```python
from build123d import *

# Parameters (mm, degrees)
BOSS_EXTRUDE1_DEPTH = 10
SKETCH2_R           = 12.5
CUT_EXTRUDE1_DEPTH  = 271.924343683
SKETCH3_R           = 7.5
CUT_EXTRUDE2_DEPTH  = 10


with BuildPart() as part:
    # Sketch1 → Boss-Extrude1 (new body)
    with BuildSketch(Plane.XY):
        with BuildLine():
            Line((-20, 0), (-20, 250))
            ThreePointArc((-20, 250), (0, 270), (20, 250))
            Line((20, 250), (20, 0))
            ThreePointArc((20, 0), (0, -20), (-20, 0))
        make_face()
    extrude(amount=BOSS_EXTRUDE1_DEPTH)

    # Sketch2 → Cut-Extrude1 (cut, through all)
    with BuildSketch(Plane(origin=(0, 0, 0), x_dir=(-1, 0, 0), z_dir=(0, 0, -1))):
        Circle(SKETCH2_R)
        with Locations((0, 250)):
            Circle(SKETCH2_R)
    extrude(amount=-CUT_EXTRUDE1_DEPTH, mode=Mode.SUBTRACT)

    # Sketch3 → Cut-Extrude2 (cut)
    with BuildSketch(Plane(origin=(0, 0, 0), x_dir=(-1, 0, 0), z_dir=(0, 0, -1))):
        with Locations((0, 125)):
            Circle(SKETCH3_R)
    extrude(amount=-CUT_EXTRUDE2_DEPTH, mode=Mode.SUBTRACT)


solid = part.part
```
Could you check a few things on this model? Use its own coordinates, in mm. Give positions to 0.01 mm unless a question says otherwise; leave off trailing zeros. Loops run counter-clockwise (first coordinate to the right, second up) from the corner with the lowest first, then second, coordinate; pieces in that order, holes last. Notation, with made-up numbers: (-12.75, 6.25) - (13.25, 6.25) arc R20 ccw to (13.25, 23.25) - close; hole circle Ø9 at (41.5, 87). An arc over 180 degrees is marked (long way). Answer in a Markdown table with one row per item. Add a question column.
Q1. If we section it at C-C (z = 5): List the corners of the cut face in (x, y) for me, plus the area to 3 significant figures.
Q2. Please list where these lines run through material, in increasing order: L1, parallel to Y at x = 0, z = 2.5; L2, parallel to Y at x = -5, z = 1.5; L3, parallel to Y at x = -9, z = 8.5. Write a range as from..to.
Q3. If we section it at B-B (y = 125): List the corners of the cut face in (x, z) for me.
Q4. For pin 1 (5 mm diameter, centred on x = 14, z = 4, fed in from +Y); pin 2 (1 mm diameter, centred on x = 11, z = 5.5, fed in from -Y); pin 3 (2 mm diameter, centred on x = 15.5, z = 6, fed in from +Y) (3 decimals), each with a flat end and sliding along its axis, tell me the tip position at first contact or that it passes through.
Q5. If we section it at A-A (x = 0): List the corners of the cut face in (y, z) for me, plus the area to 3 significant figures.
Q6. If we section it at D-D (x = -17.5): List the corners of the cut face in (y, z) for me.
Q7. We'd pull the mould along Y, two halves only. Please class faces 1 (the face through (0, -20, 5)), 2 (the face through (0, 270, 5)), 3 (the face through (-11.923, 3.755, 4.93)): +Y half, -Y half, draft (parallel to the pull), parting line (faces both ways), or undercut.
The answers:
| question | item | result |
|---|---|---|
| 1 | outline | (-20, 0) arc R20 ccw to (20, 0) - (20, 250) arc R20 ccw to (-20, 250) - close; hole circle Ø25 at (0, 0); hole circle Ø25 at (0, 250); hole circle Ø15 at (0, 125) |
| 1 | area | 10,100 mm^2 |
| 2 | L1 | y = -20..-12.5, 12.5..117.5, 132.5..237.5, 262.5..270 |
| 2 | L2 | y = -19.36..-11.46, 11.46..119.41, 130.59..238.54, 261.46..269.36 |
| 2 | L3 | y = -17.86..-8.67, 8.67..241.33, 258.67..267.86 |
| 3 | outline | (-20, 0) - (-7.5, 0) - (-7.5, 10) - (-20, 10) - close; (7.5, 0) - (20, 0) - (20, 10) - (7.5, 10) - close |
| 4 | pin 1 | stops at y = 266.36 |
| 4 | pin 2 | stops at y = -17.02 |
| 4 | pin 3 | stops at y = 263.775 |
| 5 | outline | (-20, 0) - (-12.5, 0) - (-12.5, 10) - (-20, 10) - close; (12.5, 0) - (117.5, 0) - (117.5, 10) - (12.5, 10) - close; (132.5, 0) - (237.5, 0) - (237.5, 10) - (132.5, 10) - close; (262.5, 0) - (270, 0) - (270, 10) - (262.5, 10) - close |
| 5 | area | 2,250 mm^2 |
| 6 | outline | (-9.68, 0) - (259.68, 0) - (259.68, 10) - (-9.68, 10) - close |
| 7 | face 1 | -Y half |
| 7 | face 2 | +Y half |
| 7 | face 3 | undercut |
